Source: three-view drawing plus pictorial views. Frame: mm from the lowest corner of the part. A direction names the side the tool comes from. Coordinates: 2 decimals unless noted, no trailing zeros. Order: outer loops, then holes, each group sorted by start corner. A loop starts at its lowest first (then second) coordinate and runs counter-clockwise, first axis right, second up. Notation, with made-up numbers: (72.5, 50) - (79.5, 50) arc R24 ccw to (79.5, 84) - close; hole circle Ø5 at (-21.75, 65). An arc over 180 degrees is marked (long way). One line per question, with ' | ' between items.
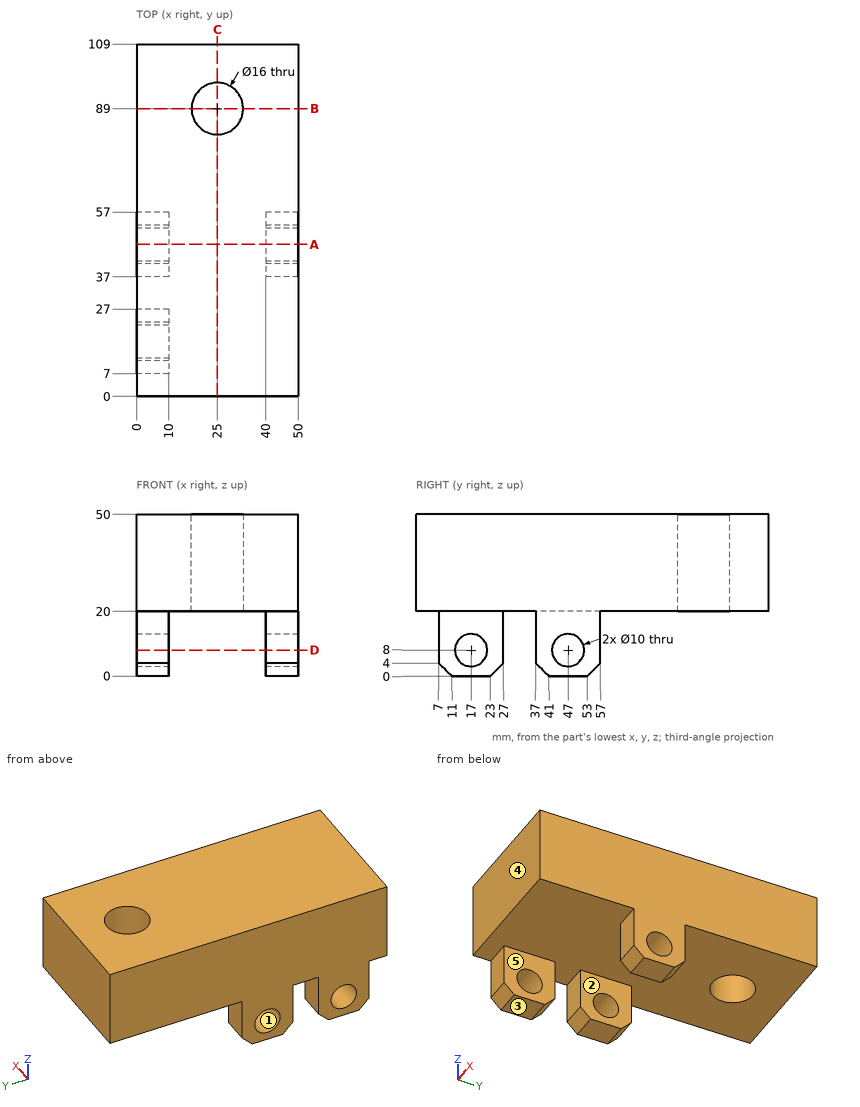
Item 1: Ray query, line 1 (Z direction, x = 42, y = 47); line 2 (Y direction, x = 25, z = 33.25); line 3 (Z direction, x = 32, y = 32). Return the intervals inside material, ascending.
Data:
line 1: 0 to 3, 13 to 50 | line 2: 0 to 81, 97 to 109 | line 3: 20 to 50
Item 2: Section D-D on z = 8. Return the cut outline in (x, y), and give its area (3 significant figures).
Data:
outline: (0, 7) - (10, 7) - (10, 12) - (0, 12) - close; (0, 22) - (10, 22) - (10, 27) - (0, 27) - close; (0, 37) - (10, 37) - (10, 42) - (0, 42) - close; (0, 52) - (10, 52) - (10, 57) - (0, 57) - close; (40, 37) - (50, 37) - (50, 42) - (40, 42) - close; (40, 52) - (50, 52) - (50, 57) - (40, 57) - close | area: 300 mm^2
Item 3: Section C-C on x = 25. Return the cut outline in (y, z).
Data:
outline: (0, 20) - (81, 20) - (81, 50) - (0, 50) - close; (97, 20) - (109, 20) - (109, 50) - (97, 50) - close
Item 4: Draft query along Z for the marked faces 1, 2 and 3. Return one class per face: released by +Z, released by -Z, zero draft, split by the parting line, or undercut.
Data:
face 1: undercut | face 2: zero draft | face 3: released by -Z
Item 5: Access query for the marked faces 4 and 5. Directions: +Z, -Z, +X, -X, +Y, -Y. A direction counts if a zero-diameter tool reaches every point of the face in a straight line with its end or side. Return the directions, or none.
Data:
face 4: +Z, -Z, +X, -X, -Y | face 5: -Z, +X, +Y, -Y
Item 6: Section A-A on y = 47. Return the cut outline in (x, z), and give its area (3 significant figures).
Data:
outline: (0, 0) - (10, 0) - (10, 3) - (0, 3) - close; (0, 13) - (10, 13) - (10, 20) - (40, 20) - (40, 13) - (50, 13) - (50, 50) - (0, 50) - close; (40, 0) - (50, 0) - (50, 3) - (40, 3) - close | area: 1,700 mm^2
Item 7: Section B-B on y = 89. Return the cut outline in (x, z), and give its area (3 significant figures).
Data:
outline: (0, 20) - (17, 20) - (17, 50) - (0, 50) - close; (33, 20) - (50, 20) - (50, 50) - (33, 50) - close | area: 1,020 mm^2
Item 8: Contact query for flat-ended pins moving along their axis: P1, Ø25, axis at x = 16, y = 76, coming from the -Z side; P2, Ø5, axis at x = 4, z = 12, coming from the -Y side; P3, Ø8, axis at y = 47, z = 8, coming from the +X side (3 decimals); P4, Ø3, axis at x = 43.5, z = 11.5, coming from the +Y side. Output: stop coordinate, or through.
Data:
P1: z = 20 | P2: y = 7 | P3: through | P4: y = 57
